The listing builds one solid part. Answer for the finished solid, in the listing's coordinates (mm). A direction names the side the tool comes from. Give positions to 0.01 mm unless a question says otherwise; leave off trailing zeros. Order: outer loops, then holes, each group sorted by start corner. A loop starts at its lowest first (then second) coordinate and runs counter-clockwise, first axis right, second up. Notation, with made-up numbers: (-11.5, 36) - (20.5, 36) arc R12 cw to (20.5, 40) - close; hole circle Ø10 at (67.5, 35.25). An arc over 180 degrees is marked (long way). Answer as a JSON object with one key per item and string values. Group by question number.
Q1. A cutting plane is placed at A-A, the plane y = 6.5. Count the separate pieces of the cut face and the enclosed holes in it, and give its area (3 significant figures).
Q2. The mould has two halves that part along X. Classify faces 3 (the face through (10.57, 5.07, -12)), 4 (the face through (49, 10, -89)), 5 (the face through (69, 6, -87.5)), 6 (the face through (138, 1, -46)): released by +X, released by -X, zero draft, split by the parting line, or undercut.
Q3. For faces 1 (the face through (69, 6, -2.5)), 2 (the face through (130.987, 5.07, -10.695)), determine the directions among +Z, -Z, +X, -X, +Y, -Y from which every point of the face is accessible in a straight line to the end or side of a thin tool.
Q4. A cutting plane is placed at B-B, the plane z = -79.5. Give the vertices of the cut face in (x, y), and give its area (3 significant figures).
Q5. A cutting plane is placed at D-D, the plane x = 42. Give the vertices of the cut face in (y, z).
Q6. A cutting plane is placed at C-C, the plane x = 10.5. Give the vertices of the cut face in (y, z).
Q7. Consider line 1 (X direction, y = 8.25, z = -79.5); line 2 (X direction, y = 7.25, z = -48); line 3 (Z direction, x = 100, y = 6.75). Determine where each line is inside the solid, lowest interval first.
Q8. Given pin 1 (5 mm diameter, centred on y = 2, z = -55.5, fed in from -X); pin 2 (1 mm diameter, centred on y = 2.5, z = -47, fed in from +X), each flat-ended and moving along its own axis, determine where each tip first touches the part or whether it passes through.
from build123d import *

# Parameters (mm, degrees)
SKETCH1_W           = 140
SKETCH1_H           = 90
BOSS_EXTRUDE2_DEPTH = 10
SKETCH2_W           = 135
SKETCH2_H           = 85
CUT_EXTRUDE1_DEPTH  = 7.5
SKETCH4_R           = 3.5
BOSS_EXTRUDE3_DEPTH = 7.5
SKETCH5_R           = 1.5
CUT_EXTRUDE2_DEPTH  = 167.733320005
FILLET1_R           = 5


with BuildPart() as part:
    # Sketch1 → Boss-Extrude2 (new body)
    with BuildSketch(Plane(origin=(0, 0, 0), x_dir=(1, 0, 0), z_dir=(0, 1, 0))):
        with Locations((70, 45)):
            Rectangle(SKETCH1_W, SKETCH1_H)
    extrude(amount=BOSS_EXTRUDE2_DEPTH)

    # Sketch2 → Cut-Extrude1 (cut)
    with BuildSketch(Plane(origin=(0, 10, 0), x_dir=(1, 0, 0), z_dir=(0, 1, 0))):
        with Locations((70, 45)):
            Rectangle(SKETCH2_W, SKETCH2_H)
    extrude(amount=-CUT_EXTRUDE1_DEPTH, mode=Mode.SUBTRACT)

    # Sketch4 → Boss-Extrude3 (add)
    with BuildSketch(Plane(origin=(0, 2.5, 0), x_dir=(1, 0, 0), z_dir=(0, 1, 0))):
        with Locations(Location((10.5, 79.5, 0), (0, 0, 270))):
            Circle(SKETCH4_R)
        with Locations(Location((10.5, 10.5, 0), (0, 0, 270))):
            Circle(SKETCH4_R)
        with Locations(Location((129.5, 10.5, 0), (0, 0, 270))):
            Circle(SKETCH4_R)
        with Locations(Location((129.5, 79.5, 0), (0, 0, 270))):
            Circle(SKETCH4_R)
    extrude(amount=BOSS_EXTRUDE3_DEPTH)

    # Sketch5 → Cut-Extrude2 (cut, through all)
    with BuildSketch(Plane(origin=(0, 10, 0), x_dir=(1, 0, 0), z_dir=(0, 1, 0))):
        with Locations(Location((10.5, 10.5, 0), (0, 0, 270))):
            Circle(SKETCH5_R)
        with Locations(Location((10.5, 79.5, 0), (0, 0, 270))):
            Circle(SKETCH5_R)
        with Locations(Location((129.5, 79.5, 0), (0, 0, 270))):
            Circle(SKETCH5_R)
        with Locations(Location((129.5, 10.5, 0), (0, 0, 270))):
            Circle(SKETCH5_R)
    extrude(amount=-CUT_EXTRUDE2_DEPTH, mode=Mode.SUBTRACT)

    # Fillet1
    fillet1_edges = [part.edges().sort_by_distance(p)[0] for p in [
        (70, 0, -90),
        (140, 0, -45),
        (70, 0, 0),
        (0, 0, -45),
    ]]
    fillet(fillet1_edges, radius=FILLET1_R)


solid = part.part
Reply:
{
 "1": {"separate pieces": "5", "enclosed holes": "5", "area": "1,250 mm^2"},
 "2": {"face 3": "undercut", "face 4": "zero draft", "face 5": "undercut", "face 6": "released by +X"},
 "3": {"face 1": "+Y", "face 2": "+Y, -Y"},
 "4": {"outline": "(0, 5) arc R5 ccw to (5, 0) - (9, 0) - (9, 10) - (7, 10) - (7, 2.5) - (2.5, 2.5) - (2.5, 10) - (0, 10) - close; (12, 0) - (128, 0) - (128, 10) - (126, 10) - (126, 2.5) - (14, 2.5) - (14, 10) - (12, 10) - close; (131, 0) - (135, 0) arc R5 ccw to (140, 5) - (140, 10) - (137.5, 10) - (137.5, 2.5) - (133, 2.5) - (133, 10) - (131, 10) - close", "area": "422 mm^2"},
 "5": {"outline": "(0, -85) arc R5 ccw to (5, -90) - (10, -90) - (10, -87.5) - (2.5, -87.5) - (2.5, -2.5) - (10, -2.5) - (10, 0) - (5, 0) arc R5 ccw to (0, -5) - close"},
 "6": {"outline": "(0, -85) arc R5 ccw to (5, -90) - (10, -90) - (10, -87.5) - (2.5, -87.5) - (2.5, -83) - (10, -83) - (10, -81) - (0, -81) - close; (0, -78) - (10, -78) - (10, -76) - (2.5, -76) - (2.5, -14) - (10, -14) - (10, -12) - (0, -12) - close; (0, -9) - (10, -9) - (10, -7) - (2.5, -7) - (2.5, -2.5) - (10, -2.5) - (10, 0) - (5, 0) arc R5 ccw to (0, -5) - close"},
 "7": {"line 1": "x = 0 to 2.5, 7 to 9, 12 to 14, 126 to 128, 131 to 133, 137.5 to 140", "line 2": "x = 0 to 2.5, 137.5 to 140", "line 3": "z = -90 to -87.5, -2.5 to 0"},
 "8": {"pin 1": "stops at x = 0.03", "pin 2": "stops at x = 139.58"}
}
